Source: CAD feature listing. Evaluate the final solid. Frame: model axes, mm. A direction names the side the tool comes from. Round coordinates to 2 decimals unless told otherwise and drop trailing zeros. Write each loop counter-clockwise with the first axis right and the second up, starting at its lowest first coordinate (ties: lowest second). Pieces come first, ordered by that corner, then holes. Notation, with made-up numbers: M 57,18.25 L 101,18.25 A21 ccw 101,49.25 Z; hole C -17,71.25 d5. An arc over 180 degrees is marked long. Put each result on its own line as item: value. Start each with the question number.
```python
from build123d import *

# Parameters (mm, degrees)
SKETCH2_W           = 10
SKETCH2_H           = 10
SKETCH3_R           = 10
BOSS_EXTRUDE1_DEPTH = 10


with BuildPart() as part:
    # Sketch2 → Revolve1 (revolve)
    with BuildSketch(Plane.XY):
        with Locations((0, 5)):
            Rectangle(SKETCH2_W, SKETCH2_H)
        with BuildLine():
            Line((-5, 50), (-5, 10))
            Line((-5, 10), (5, 10))
            ThreePointArc((5, 10), (6.128537222, 30.126164563), (9.5, 50))
            Line((9.5, 50), (10, 50))
            ThreePointArc((10, 50), (2.5, 57.5), (-5, 50))
        make_face()
    revolve(axis=Axis((-5, 0, 0), (1, 0, 0)))

    # Sketch3 → Boss-Extrude1 (add)
    with BuildSketch(Plane.ZY.offset(5)):
        Circle(SKETCH3_R)
    extrude(amount=BOSS_EXTRUDE1_DEPTH)


solid = part.part
```
(1) Section query B-B (x = 0.25). Return loops of the section in (y, z), and give its area (3 significant figures).
(2) Section query A-A (x = -11). Return loops of the section in (y, z).
(3) Ray query, line 1 along X through (y, z) = (50, 2.5); line 2 along Y through (x, z) = (-2.5, -27.5); line 3 along Z through (x, y) = (-11.5, 2). Return the intervals inside material, ascending.
(4) Contact query for flat-ended pins moving along their axis: P1, Ø10, axis at y = -3.5, z = -3.5, coming from the +X side; P2, Ø6, axis at x = -2, z = -14.5, coming from the +Y side; P3, Ø5, axis at x = -2.5, z = 43, coming from the +Y side. Output: stop coordinate, or through.
(5) Access query for faces 4 (the flat face through (-15, 0, 0)), 5 (the flat face through (5, 0, 0)). Directions: +Z, -Z, +X, -X, +Y, -Y. A direction counts if a zero-diameter tool reaches every point of the face in a straight line with its end or side. Return the directions, or none.
(6) Pull-direction query (Z, two-part tool) for faces 1 (the flat face through (-5, -0.7, -10.4)), 2 (the cylindrical face through (-9.93, -9.76, -2.17)), 3 (the cylindrical face through (9.75, 47.69, 15.02)); classes: +Z half, -Z half, draft (parallel to the pull), parting line (faces both ways), or undercut.
Entries:
1. outline: C 0,0 d114.31
1. area: 10,300 mm2
2. outline: C 0,0 d20
3. line 1: -5 to 10
3. line 2: -48.31 to 48.31
3. line 3: -9.8 to 9.8
4. P1: x = 5
4. P2: y = 55.77
4. P3: y = 39.07
5. face 4: +Z, -Z, -X, +Y, -Y
5. face 5: +X
6. face 1: draft
6. face 2: parting line
6. face 3: undercut
